Work out the finished part from the listing and answer in its coordinate system (mm). Round coordinates to 2 decimals unless told otherwise and drop trailing zeros. Write each loop counter-clockwise with the first axis right and the second up, starting at its lowest first coordinate (ties: lowest second). Pieces come first, ordered by that corner, then holes. Notation, with made-up numbers: (51, 51.25) - (68, 51.25) arc R35 ccw to (68, 83.25) - close; hole circle Ø1 at (-4.5, -0.75). An arc over 180 degrees is marked (long way). Answer as a JSON object with one key per item and string values.
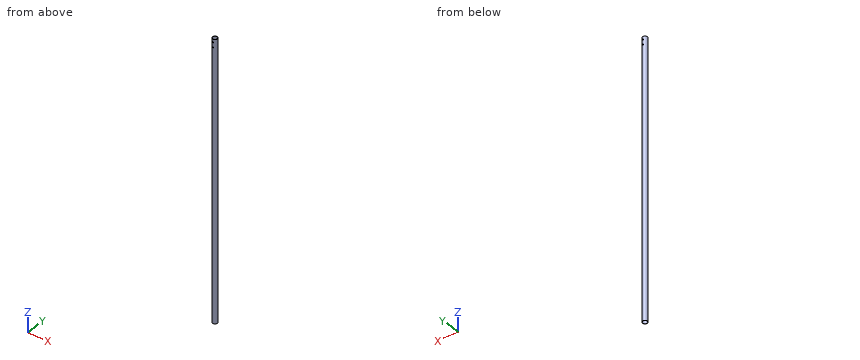
```python
from build123d import *

# Parameters (mm, degrees)
SKETCH2_R                     = 12.7
SKETCH2_R_2                   = 11.1125
BOSS_EXTRUDE1_DEPTH           = 1400
SKETCH6_W                     = 2.75
SKETCH6_H                     = 12.7
M5_CLEARANCE_HOLE1_AT_2_COUNT = 2
M5_CLEARANCE_HOLE1_AT_2_PITCH = 25
MIRROR1_COPY_1_SKETCH_W       = 2.75
MIRROR1_COPY_1_SKETCH_H       = 12.7


with BuildPart() as part:
    # Sketch2 → Boss-Extrude1 (new body)
    with BuildSketch(Plane.XY):
        Circle(SKETCH2_R)
        Circle(SKETCH2_R_2, mode=Mode.SUBTRACT)
    extrude(amount=BOSS_EXTRUDE1_DEPTH)

    # Sketch6 → M5 Clearance Hole1 (revolve, cut)
    with BuildSketch(Plane(origin=(0, 0, 1385), x_dir=(0, 0, -1), z_dir=(1, 0, 0))):
        with Locations((1.375, 6.35)):
            Rectangle(SKETCH6_W, SKETCH6_H)
    m5_clearance_hole1 = revolve(axis=Axis((0, -6.35, 1385), (0, 1, 0)), mode=Mode.SUBTRACT)

    # M5 Clearance Hole1 at 2: M5 Clearance Hole1 ×2
    with Locations(*[(0, 0, -i * M5_CLEARANCE_HOLE1_AT_2_PITCH) for i in range(1, M5_CLEARANCE_HOLE1_AT_2_COUNT)]):
        add(m5_clearance_hole1, mode=Mode.SUBTRACT)

    # Mirror1: M5 Clearance Hole1 across plane
    add(m5_clearance_hole1.mirror(Plane.ZX), mode=Mode.SUBTRACT)

    # Mirror1 copy 1 sketch → Mirror1 copy 1 (revolve, cut)
    with BuildSketch(Plane(origin=(0, 0, 1360), x_dir=(0, 0, -1), z_dir=(1, 0, 0))):
        with Locations((1.375, -6.35)):
            Rectangle(MIRROR1_COPY_1_SKETCH_W, MIRROR1_COPY_1_SKETCH_H)
    revolve(axis=Axis((0, 6.35, 1360), (0, 1, 0)), mode=Mode.SUBTRACT)


solid = part.part
```
Item 1: A cutting plane is placed at B-B (z = 1289.5). Write down the section's boundary in (x, y) (1 decimal).
Results found:
{"outline": "circle Ø25.4 at (0, 0); hole circle Ø22.2 at (0, 0)"}
Item 2: A cutting plane is placed at A-A (y = 0). Write down the section's boundary in (x, z).
Results found:
{"outline": "(-12.7, 0) - (-11.11, 0) - (-11.11, 1400) - (-12.7, 1400) - close; (11.11, 0) - (12.7, 0) - (12.7, 1400) - (11.11, 1400) - close"}
Item 3: Each of these flat-tipped pins is pushed along its axis until it touches: P1, Ø1, axis at x = -8, z = 326.5, coming from the +Y side; P2, Ø3, axis at y = 2.5, z = 384.5, coming from the -X side; P3, Ø1, axis at y = -6.5, z = 1186, coming from the +X side. Where does it stop, or does it pass through?
Results found:
{"P1": "y = 10.25", "P2": "x = -12.66", "P3": "x = 11.19"}
Item 4: Consider line 1 along Z through (x, y) = (0.25, -11.25); line 2 along Y through (x, z) = (-2.5, 1082.5); line 3 along Y through (x, z) = (0, 133). Determine where each line is inside the solid, lowest interval first.
Results found:
{"line 1": "0 to 1357.26, 1362.74 to 1382.26, 1387.74 to 1400", "line 2": "-12.45 to -10.83, 10.83 to 12.45", "line 3": "-12.7 to -11.11, 11.11 to 12.7"}
